Here's how the part is built. I have some questions about the finished solid (model axes, mm). Face numbers are marked on the shaded views. A direction names the side the tool comes from. Give positions to 0.01 mm unless a question says otherwise; leave off trailing zeros. Write each loop counter-clockwise with the first axis right and the second up, starting at its lowest first coordinate (ties: lowest second). Pieces come first, ordered by that corner, then holes. Notation, with made-up numbers: M -3,72 L 1,72 A21 cw 1,92 Z; hole C 68,21 d5. An arc over 180 degrees is marked long. Answer as CSV lines item,"result". Start each with the question number.
Q1. Suppose I cut it at B-B (z = 8.75). Write out the boundary of the cut face in (x, y), then the cut area to 3 significant figures.
Q2. Suppose I cut it at A-A (y = 0). Write out the boundary of the cut face in (x, z), then the cut area to 3 significant figures.
Q3. On a 3-axis mill with a long thin cutter (end or side, diameter ignored), from which of +Z, -Z, +X, -X, +Y, -Y can I reach the whole of each face in a straight line? I mean the marked faces 1 and 2. Say none if no direction works.
Q4. For pin 1 (2 mm diameter, centred on x = 9, y = -6, fed in from -Z), with a flat end and sliding along its axis, tell me the tip position at first contact or that it passes through.
Q5. Thinking about a two-plate mould opening in X: for the marked faces 3, 4 and 5, which applies, +X half, -X half, draft (parallel to the pull), parting line (faces both ways), or undercut?
Q6. Suppose I cut it at D-D (z = 4). Write out the boundary of the cut face in (x, y).
Q7. If I drill on line 1 along Y through (x, z) = (0, 2.25); line 2 along Z through (x, y) = (11.75, -1.5); line 3 along X through (y, z) = (7.5, 2), over which ranges is the centre line in solid material (lowest first)?
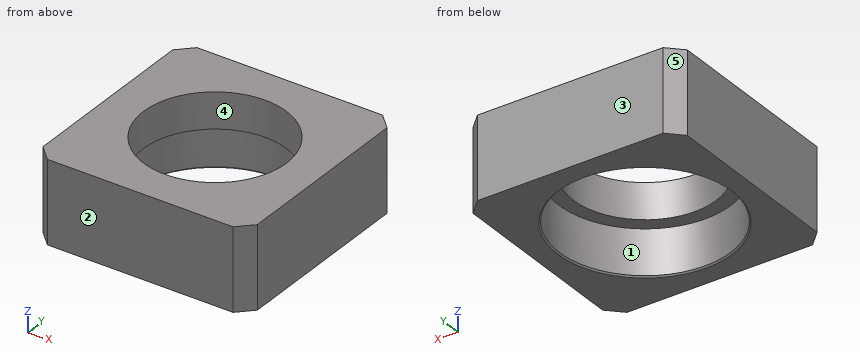
```python
from build123d import *

# Parameters (mm, degrees)
SKETCH1_W           = 30
SKETCH1_H           = 30
BOSS_EXTRUDE1_DEPTH = 11.5
SKETCH2_R           = 12
CUT_EXTRUDE1_DEPTH  = 6.5
SKETCH3_R           = 10
CUT_EXTRUDE2_DEPTH  = 6
CHAMFER1_SIZE       = 2
CHAMFER_1_SIZE      = 0.2


with BuildPart() as part:
    # Sketch1 → Boss-Extrude1 (new body)
    with BuildSketch(Plane.XY):
        Rectangle(SKETCH1_W, SKETCH1_H)
    extrude(amount=BOSS_EXTRUDE1_DEPTH)

    # Sketch2 → Cut-Extrude1 (cut)
    with BuildSketch(Plane(origin=(0, 0, 0), x_dir=(-1, 0, 0), z_dir=(0, 0, -1))):
        Circle(SKETCH2_R)
    extrude(amount=-CUT_EXTRUDE1_DEPTH, mode=Mode.SUBTRACT)

    # Sketch3 → Cut-Extrude2 (cut, through all)
    with BuildSketch(Plane(origin=(0, 0, 6.5), x_dir=(-1, 0, 0), z_dir=(0, 0, -1))):
        Circle(SKETCH3_R)
    extrude(amount=-CUT_EXTRUDE2_DEPTH, mode=Mode.SUBTRACT)

    # Chamfer1
    chamfer1_edges = [part.edges().sort_by_distance(p)[0] for p in [
        (-15, -15, 5.75),
        (-15, 15, 5.75),
        (15, 15, 5.75),
        (15, -15, 5.75),
    ]]
    chamfer(chamfer1_edges, length=CHAMFER1_SIZE)

    # 倒角1
    chamfer_1_edges = [part.edges().sort_by_distance(p)[0] for p in [
        (12, 0, 0),
    ]]
    chamfer(chamfer_1_edges, length=CHAMFER_1_SIZE)


solid = part.part
```
Resolved:
1,outline,"M -15,-13 L -13,-15 L 13,-15 L 15,-13 L 15,13 L 13,15 L -13,15 L -15,13 Z; hole C 0,0 d20"
1,area,"578 mm^2"
2,outline,"M -15,0 L -12.2,0 L -12,0.2 L -12,6.5 L -10,6.5 L -10,11.5 L -15,11.5 Z; M 10,6.5 L 12,6.5 L 12,0.2 L 12.2,0 L 15,0 L 15,11.5 L 10,11.5 Z"
2,area,"89.0 mm^2"
3,face 1,"-Z"
3,face 2,"+Z, -Z, +X, -X, -Y"
4,pin 1,"z = 6.5"
5,face 3,"draft"
5,face 4,"undercut"
5,face 5,"-X half"
6,outline,"M -15,-13 L -13,-15 L 13,-15 L 15,-13 L 15,13 L 13,15 L -13,15 L -15,13 Z; hole C 0,0 d24"
7,line 1,"-15 to -12, 12 to 15"
7,line 2,"6.5 to 11.5"
7,line 3,"-15 to -9.37, 9.37 to 15"
